Can you work these out from the model? Positions are in its coordinate system, mm. Face numbers are marked on the shaded views. A direction names the side the tool comes from. Coordinates: 2 decimals unless noted, no trailing zeros. Loops run counter-clockwise (first coordinate to the right, second up) from the corner with the lowest first, then second, coordinate; pieces in that order, holes last.
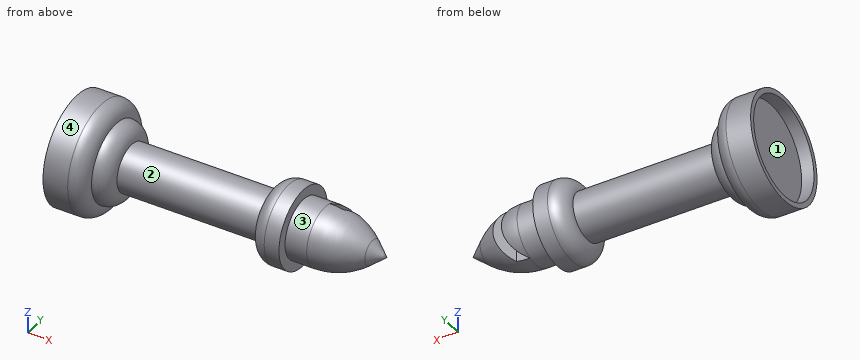
```python
from build123d import *

# Parameters (mm, degrees)
CUT_EXTRUDE_1_DEPTH = 10
SKETCH_5_R          = 10
CUT_EXTRUDE_2_DEPTH = 2.5


with BuildPart() as part:
    # Эскиз1 → Повернуть1 (revolve)
    with BuildSketch(Plane.XY, mode=Mode.PRIVATE) as revolve_1_sk:
        Polygon((5, 11), (0, 11), (0, 0), (5, 0), (5, 3), align=None)
        Polygon((8, 11), (5, 11), (5, 3), (8, 3), (8, 6.2), align=None)
        with BuildLine():
            Line((8, 3), (5, 3))
            Line((5, 3), (5, 0))
            ThreePointArc((5, 0), (7.121320344, 0.878679656), (8, 3))
        make_face()
        with BuildLine():
            Line((11.2, 6.2), (8, 6.2))
            Line((8, 6.2), (8, 3))
            ThreePointArc((8, 3), (10.2627417, 3.9372583), (11.2, 6.2))
        make_face()
        Polygon((43, 11), (8, 11), (8, 6.2), (11.2, 6.2), (39.8, 6.2), (43, 6.2), align=None)
        with BuildLine():
            Line((43, 3), (43, 6.2))
            Line((43, 6.2), (39.8, 6.2))
            ThreePointArc((39.8, 6.2), (40.7372583, 3.9372583), (43, 3))
        make_face()
        Polygon((46, 11), (43, 11), (43, 6.2), (43, 3), (46, 3), (46, 5), (46, 9), align=None)
        with BuildLine():
            Line((63, 11), (46, 11))
            Line((46, 11), (46, 9))
            Line((46, 9), (46, 5))
            Line((46, 5), (50.38992493, 5))
            ThreePointArc((50.38992493, 5), (55.52022708, 5.904610688), (60.031739076, 8.509333353))
            Line((60.031739076, 8.509333353), (63, 11))
        make_face()
    revolve(revolve_1_sk.sketch.rotate(Axis((0, 11, 0), (1, 0, 0)), 270), axis=Axis((0, 11, 0), (1, 0, 0)))

    # Эскиз2 → Вырез-Вытянуть1 (cut)
    with BuildSketch(Plane.XY):
        Polygon((50.38992493, 12.688629435), (54.167703604, 17), (55.999437229, 15.951404954), (53.140475424, 12.688629435), align=None)
    cut_extrude_1 = extrude(amount=-CUT_EXTRUDE_1_DEPTH, mode=Mode.SUBTRACT)

    # Зеркальное отражение1: Вырез-Вытянуть1 across plane
    add(cut_extrude_1.mirror(Plane.XY), mode=Mode.SUBTRACT)

    # Эскиз5 → Вырез-Вытянуть2 (cut)
    with BuildSketch(Plane.ZY):
        with Locations((0, 11)):
            Circle(SKETCH_5_R)
    extrude(amount=-CUT_EXTRUDE_2_DEPTH, mode=Mode.SUBTRACT)


solid = part.part
```
Item 1: I'm going to push flat-ended pins straight in: P1, Ø6, axis at y = 5.5, z = -7.5, coming from the +X side; P2, Ø8, axis at y = 16.5, z = -5.5, coming from the +X side; P3, Ø2, axis at x = 35, y = 7, coming from the +Z side. Where does each tip first touch, or does it pass through?
Results are:
P1: stops at x = 46
P2: stops at x = 58.25
P3: stops at z = 3.75
Item 2: We'd pull the mould along Z, two halves only. Please class the marked faces 1 and 2: +Z half, -Z half, draft (parallel to the pull), parting line (faces both ways), or undercut.
Results are:
face 1: undercut
face 2: parting line
Item 3: Suppose I cut it at A-A, the plane x = 13.5. Please give me the cut outline in (y, z).
Results are:
outline: circle Ø9.6 at (11, 0)
Item 4: I need wall thicknesses on line 1 along Y through (x, z) = (1.6, 0); line 2 along X through (y, z) = (14.5, -7.25); line 3 along Z through (x, y) = (52.5, 16.25). Which ranges of each line are inside material? Lowest first, please.
Results are:
line 1: y = 0 to 1, 21 to 22
line 2: x = 2.5 to 8
line 3: z = -2.58 to 2.58
Item 5: On a 3-axis mill with a long thin cutter (end or side, diameter ignored), from which of +Z, -Z, +X, -X, +Y, -Y can I reach the whole of each face in a straight line? I mean the marked faces 3 and 4. Say none if no direction works.
Results are:
face 3: +X
face 4: +X, -X
